Work out the finished part from the listing and answer in its coordinate system (mm). A direction names the side the tool comes from. Round coordinates to 2 decimals unless told otherwise and drop trailing zeros. Loops run counter-clockwise (first coordinate to the right, second up) from the corner with the lowest first, then second, coordinate; pieces in that order, holes last. Notation, with made-up numbers: (18.5, 85.5) -> (26.5, 85.5) arc R35 ccw to (26.5, 122.5) -> close; hole circle Ø6 at (77.5, 6.5). An arc over 180 degrees is marked (long way). Use one line per item in the form item = value.
```python
from build123d import *

# Parameters (mm, degrees)
F0_R      = 5
F1_DEPTH  = 10
F2_R      = 5
F3_DEPTH  = 25
F3_FACE_R = 5
F4_DEPTH  = 15


with BuildPart() as f1:
    # F0 (on Top) → F1 (new body, symmetric)
    with BuildSketch(Plane.XY):
        with BuildLine():
            Line((-10, -25), (10, -25))
            Line((10, -25), (10, 25))
            ThreePointArc((10, 25), (0, 35), (-10, 25))
            Line((-10, 25), (-10, -25))
        make_face()
        with Locations((0, 25)):
            Circle(F0_R, mode=Mode.SUBTRACT)
    extrude(amount=F1_DEPTH, both=True)

    # F2 (on Top) → F3 (join, symmetric)
    with BuildSketch(Plane.XY):
        with Locations((0, 25)):
            Circle(F2_R)
    extrude(amount=F3_DEPTH, both=True)

    # F3_face (on face) → F4 (cut)
    with BuildSketch(Plane(origin=(0, 25, -25), x_dir=(1, 0, 0), z_dir=(0, 0, -1))):
        Circle(F3_FACE_R)
    extrude(amount=-F4_DEPTH, mode=Mode.SUBTRACT)


solid = f1.part
```
(1) Given P1, Ø5, axis at x = 8, y = 22.5, coming from the +Z side; P2, Ø2, axis at y = 23.5, z = 13, coming from the -X side, each flat-ended and moving along its own axis, determine where each tip first touches the part or whether it passes through.
Completed:
P1 = 10
P2 = -4.97
(2) Find section C-C, the plane z = 14. Write down the section's boundary in (x, y), then the cut area to 3 significant figures.
Completed:
outline = circle Ø10 at (0, 25)
area = 78.5 mm2
(3) Find section B-B, the plane y = -18.5. Write down the section's boundary in (x, z), then the cut area to 3 significant figures.
Completed:
outline = (-10, -10) -> (10, -10) -> (10, 10) -> (-10, 10) -> close
area = 400 mm2
(4) For faces 1 (the flat face through (0, 5, -10)), 2 (the cylindrical face through (-1.08, 20.12, 17.6)), determine the directions among +Z, -Z, +X, -X, +Y, -Y from which every point of the face is accessible in a straight line to the end or side of a thin tool.
Completed:
face_1 = -Z, +X, -X, +Y, -Y
face_2 = +Z
(5) Find section D-D, the plane x = 3.25. Write down the section's boundary in (y, z).
Completed:
outline = (-25, -10) -> (34.46, -10) -> (34.46, 10) -> (28.8, 10) -> (28.8, 25) -> (21.2, 25) -> (21.2, 10) -> (-25, 10) -> close
(6) Find section A-A, the plane x = 0. Write down the section's boundary in (y, z).
Completed:
outline = (-25, -10) -> (35, -10) -> (35, 10) -> (30, 10) -> (30, 25) -> (20, 25) -> (20, 10) -> (-25, 10) -> close
(7) Consider L1, parallel to Y at x = 0, z = -0.5; L2, parallel to Z at x = 8.75, y = -6; L3, parallel to Y at x = -0.25, z = 17. Determine where each line is inside the solid, lowest interval first.
Completed:
L1 = -25 to 35
L2 = -10 to 10
L3 = 20.01 to 29.99
